Here's how the part is built. I have some questions about the finished solid (model axes, mm). Round coordinates to 2 decimals unless told otherwise and drop trailing zeros. Loops run counter-clockwise (first coordinate to the right, second up) from the corner with the lowest first, then second, coordinate; pieces in that order, holes last. Notation, with made-up numbers: M 37.5,35 L 49.5,35 A24 ccw 49.5,57 Z; hole C 2.25,35.25 d8. An arc over 180 degrees is marked long. Answer as a JSON object with one key per item and string values.
from build123d import *

# Parameters (mm, degrees)
SKETCH1_R           = 2.0193
SKETCH1_R_2         = 14.2875
BOSS_EXTRUDE1_DEPTH = 1.5875


with BuildPart() as part:
    # Sketch1 → Boss-Extrude1 (new body)
    with BuildSketch(Plane(origin=(0, 0, 0), x_dir=(0, 0, -1), z_dir=(1, 0, 0))):
        with BuildLine():
            Line((288.401681083, 160.383356591), (249.345231223, 146.9200509))
            Line((249.345231223, 146.9200509), (266.935398847, 95.891758474))
            Line((266.935398847, 95.891758474), (296.387053498, 106.044156633))
            Line((296.387053498, 106.044156633), (331.100032982, 91.851270852))
            Line((331.100032982, 91.851270852), (351.527026912, 141.811640586))
            Line((351.527026912, 141.811640586), (307.41026186, 159.849395245))
            ThreePointArc((307.41026186, 159.849395245), (297.954559489, 161.846069046), (288.401681083, 160.383356591))
        make_face()
        with Locations((269.613187196, 132.077455087)):
            Circle(SKETCH1_R, mode=Mode.SUBTRACT)
        with Locations((271.682618681, 126.074126566)):
            Circle(SKETCH1_R, mode=Mode.SUBTRACT)
        with Locations((273.752050167, 120.070798045)):
            Circle(SKETCH1_R, mode=Mode.SUBTRACT)
        with Locations((297.196764895, 134.869210378)):
            Circle(SKETCH1_R_2, mode=Mode.SUBTRACT)
        with Locations((324.580125518, 130.53340397)):
            Circle(SKETCH1_R, mode=Mode.SUBTRACT)
        with Locations((322.176949762, 124.655713413)):
            Circle(SKETCH1_R, mode=Mode.SUBTRACT)
        with Locations((319.773774005, 118.778022856)):
            Circle(SKETCH1_R, mode=Mode.SUBTRACT)
    extrude(amount=-BOSS_EXTRUDE1_DEPTH)


solid = part.part
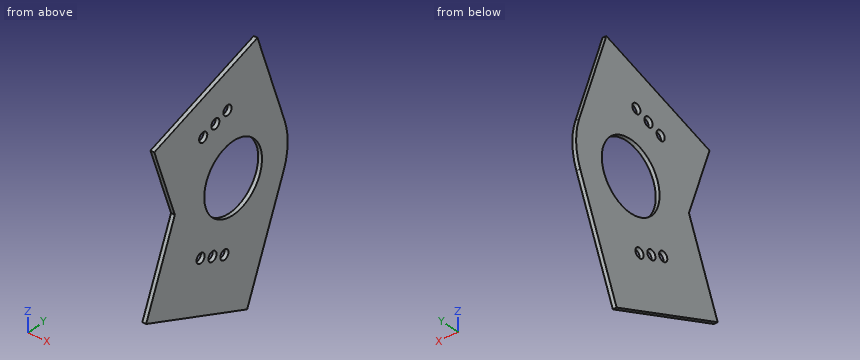
Item 1: I want a section at B-B, the plane y = 145.5. Please give me the cut outline in (x, z).
Resolved:
{"outline": "M -1.59,-342.51 L 0,-342.51 L 0,-306.74 L -1.59,-306.74 Z; M -1.59,-287.65 L 0,-287.65 L 0,-249.83 L -1.59,-249.83 Z"}
Item 2: I'm going to push a flat-ended pin straight in: pin 1 Ø3.5 at (y, z) = (130.53, -324.58) entering from +X (3 decimals). Where does the tip first touch, or does it pass through?
Resolved:
{"pin 1": "through"}
Item 3: I want a section at A-A, the plane z = -310. Please give me the cut outline in (x, y), then the cut area to 3 significant figures.
Resolved:
{"outline": "M -1.59,100.48 L 0,100.48 L 0,128.53 L -1.59,128.53 Z; M -1.59,141.21 L 0,141.21 L 0,158.79 L -1.59,158.79 Z", "area": "72.4 mm²"}
Item 4: Please list where these lines run through material, in increasing order: probe 1 along Y at (x, z) = (-1.15, -321); probe 2 along Z at (x, y) = (-1, 124); probe 3 along Z at (x, y) = (-1, 142). Write a range as from..to.
Resolved:
{"probe 1": "95.98..117.17, 120.38..123.01, 126.3..154.29", "probe 2": "-344.24..-324.09, -320.27..-306.47, -287.92..-257.25", "probe 3": "-351.07..-309.58, -284.82..-251.04"}
Item 5: I want a section at C-C, the plane x = -0.3. Please give me the cut outline in (y, z) (1 decimal), then the cut area to 3 significant figures.
Resolved:
{"outline": "M 91.9,-331.1 L 141.8,-351.5 L 159.8,-307.4 A27 ccw 160.4,-288.4 L 146.9,-249.3 L 95.9,-266.9 L 106,-296.4 Z; hole C 118.8,-319.8 d4; hole C 120.1,-273.8 d4; hole C 134.9,-297.2 d28.6; hole C 124.7,-322.2 d4; hole C 126.1,-271.7 d4; hole C 130.5,-324.6 d4; hole C 132.1,-269.6 d4", "area": "4,070 mm²"}
Item 6: I want a section at D-D, the plane y = 155.5. Please give me the cut outline in (x, z), then the cut area to 3 significant figures.
Resolved:
{"outline": "M -1.59,-318.05 L 0,-318.05 L 0,-274.24 L -1.59,-274.24 Z", "area": "69.6 mm²"}
